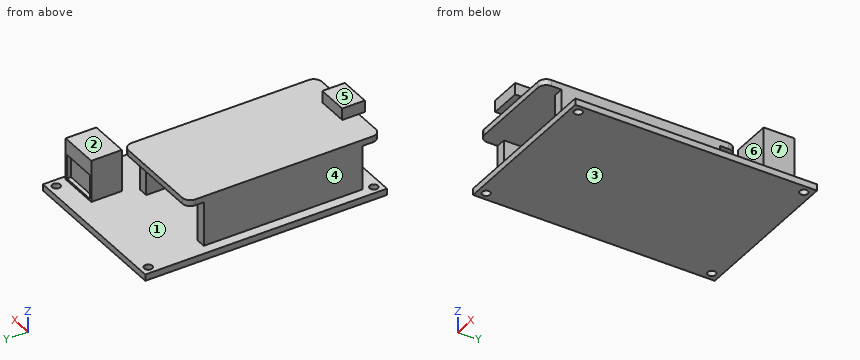
from build123d import *

# Parameters (mm, degrees)
F0_W      = 40
F0_H      = 60
F0_R      = 1
F1_DEPTH  = 1.6
F2_W      = 10
F2_H      = 7.6
F3_DEPTH  = 10.4
F4_W      = 9
F4_H      = 6
F5_DEPTH  = 1
F6_W      = 2.5
F6_H      = 39.4
F7_DEPTH  = 11
F8_W      = 25
F8_H      = 48
F9_DEPTH  = 1.5
F10_R     = 2
F11_W     = 7.8
F11_H     = 5.6
F12_DEPTH = 2.9


with BuildPart() as f1:
    # F0 (on Top) → F1 (new body)
    with BuildSketch(Plane.XY):
        Rectangle(F0_W, F0_H)
        with Locations((-18, -28)):
            Circle(F0_R, mode=Mode.SUBTRACT)
        with Locations((18, -28)):
            Circle(F0_R, mode=Mode.SUBTRACT)
        with Locations((-18, 28)):
            Circle(F0_R, mode=Mode.SUBTRACT)
        with Locations((18, 28)):
            Circle(F0_R, mode=Mode.SUBTRACT)
    extrude(amount=F1_DEPTH)

    # F2 (on face) → F3 (join)
    with BuildSketch(Plane.XY.offset(1.6)):
        with Locations((14, 21.2)):
            Rectangle(F2_W, F2_H)
    extrude(amount=F3_DEPTH)

    # F4 (on face) → F5 (cut)
    with BuildSketch(Plane(origin=(0, 25, 0), x_dir=(-1, 0, 0), z_dir=(0, 1, 0))):
        with Locations((-14, 5.1)):
            Rectangle(F4_W, F4_H)
    extrude(amount=-F5_DEPTH, mode=Mode.SUBTRACT)

    # F6 (on face) → F7 (join)
    with BuildSketch(Plane.XY.offset(1.6)):
        with Locations((6.25, -5.8)):
            Rectangle(F6_W, F6_H)
        with Locations((-16.25, -5.8)):
            Rectangle(F6_W, F6_H)
    extrude(amount=F7_DEPTH)

    # F8 (on face) → F9 (join)
    with BuildSketch(Plane.XY.offset(12.6)):
        with Locations((-5, -6.032404)):
            Rectangle(F8_W, F8_H)
    extrude(amount=F9_DEPTH)

    # F10
    f10_edges = [f1.edges().sort_by_distance(p)[0] for p in [
        (-17.5, -30.032404, 13.35),
        (7.5, -30.032404, 13.35),
        (7.5, 17.967596, 13.35),
        (-17.5, 17.967596, 13.35),
    ]]
    fillet(f10_edges, radius=F10_R)

    # F11 (on face) → F12 (join)
    with BuildSketch(Plane.XY.offset(14.1)):
        with Locations((-5, -28.732404)):
            Rectangle(F11_W, F11_H)
    extrude(amount=F12_DEPTH)


solid = f1.part
Can you work these out from the model? Positions are in its coordinate system, mm. Face numbers are marked on the shaded views. A direction names the side the tool comes from. Coordinates: 2 decimals unless noted, no trailing zeros. Write each loop counter-clockwise with the first axis right and the second up, starting at its lowest first coordinate (ties: lowest second). Pieces come first, ordered by that corner, then holes.
Q1. Imagine slicing it at A-A, the plane y = 28. List the corners of the cut face in (x, z) for me.
Results found:
outline: (-20, 0) - (-19, 0) - (-19, 1.6) - (-20, 1.6) - close; (-17, 0) - (17, 0) - (17, 1.6) - (-17, 1.6) - close; (19, 0) - (20, 0) - (20, 1.6) - (19, 1.6) - close
Q2. Imagine slicing it at D-D, the plane y = -24. List the corners of the cut face in (x, z) for me.
Results found:
outline: (-20, 0) - (20, 0) - (20, 1.6) - (7.5, 1.6) - (7.5, 14.1) - (-17.5, 14.1) - (-17.5, 1.6) - (-20, 1.6) - close; hole (-15, 1.6) - (5, 1.6) - (5, 12.6) - (-15, 12.6) - close
Q3. If we mould it in two halves opening along Z, with no side actions, what happens to the marked faces 1, 2 and 3? For each: +Z half, -Z half, draft (parallel to the pull), parting line (faces both ways), or undercut.
Results found:
face 1: undercut
face 2: +Z half
face 3: -Z half
Q4. Imagine slicing it at B-B, the plane x = -4. List the corners of the cut face in (y, z) for me.
Results found:
outline: (-31.53, 14.1) - (-30.03, 14.1) - (-30.03, 12.6) - (17.97, 12.6) - (17.97, 14.1) - (-25.93, 14.1) - (-25.93, 17) - (-31.53, 17) - close; (-30, 0) - (30, 0) - (30, 1.6) - (-30, 1.6) - close
Q5. Imagine slicing it at C-C, the plane x = 11.5. List the corners of the cut face in (y, z) for me.
Results found:
outline: (-30, 0) - (30, 0) - (30, 1.6) - (25, 1.6) - (25, 2.1) - (24, 2.1) - (24, 8.1) - (25, 8.1) - (25, 12) - (17.4, 12) - (17.4, 1.6) - (-30, 1.6) - close
Q6. For P1, Ø1.2, axis at x = -16, z = 9, coming from the +Y side; P2, Ø1.6, axis at x = -3.5, z = 13.5, coming from the +Y side; P3, Ø3, axis at y = -27.5, z = 16.5, coming from the +X side, each with a flat end and sliding along its axis, tell me the tip position at first contact or that it passes through.
Results found:
P1: stops at y = 13.9
P2: stops at y = 17.97
P3: stops at x = -1.1
Q7. Which directions (+Z, -Z, +X, -X, +Y, -Y) give clear straight access to the entire face, cutting with the end or side of a thin tool? Please do the marked faces 4, 5, 6 and 7.
Results found:
face 4: +Z, -X, +Y, -Y
face 5: +Z, +X, -X, +Y, -Y
face 6: +Z, +X, -X, -Y
face 7: +Z, +X, +Y, -Y
Q8. Please list where these lines run through material, in increasing order: L1, parallel to Y at x = -18, z = 1; L2, parallel to Z at x = -4, y = -27.5; L3, parallel to X at y = -10, z = 10.5.
Results found:
L1: y = -30 to -29, -27 to 27, 29 to 30
L2: z = 0 to 1.6, 12.6 to 17
L3: x = -17.5 to -15, 5 to 7.5
